Model file for the job. Use its own axes, mm. Give positions to 0.01 mm unless a question says otherwise; leave off trailing zeros. Loops run counter-clockwise (first coordinate to the right, second up) from the corner with the lowest first, then second, coordinate; pieces in that order, holes last. Notation, with made-up numbers: M 65.5,57.5 L 78.5,57.5 A31 cw 78.5,96.5 Z; hole C 46.5,30.5 d8. An arc over 180 degrees is marked long. Answer in a Markdown table with one row per item.
```python
from build123d import *

# Parameters (mm, degrees)
BOSS_EXTRUDE1_DEPTH = 9.3
SKETCH2_W           = 35
SKETCH2_H           = 6
BOSS_EXTRUDE2_DEPTH = 9.3


with BuildPart() as part:
    # Sketch1 → Boss-Extrude1 (new body)
    with BuildSketch(Plane.XY):
        Polygon((0, 0), (0, 42), (-10, 42), (-35, 2), (-35, 0), align=None)
    extrude(amount=-BOSS_EXTRUDE1_DEPTH)

    # Sketch2 → Boss-Extrude2 (add)
    with BuildSketch(Plane.XY):
        with Locations((-17.5, -3)):
            Rectangle(SKETCH2_W, SKETCH2_H)
    extrude(amount=-BOSS_EXTRUDE2_DEPTH)


solid = part.part
```
Q1. Saw through at A-A (z = -6.5). Give the cut face in (x, y).
Reported:
| item | result |
|---|---|
| outline | M -35,-6 L 0,-6 L 0,42 L -10,42 L -35,2 Z |
Q2. Drop flat-ended pins along their axis: pin 1 (4 mm diameter, centred on y = 31, z = -5.5, fed in from -X) (3 decimals); pin 2 (1.5 mm diameter, centred on x = -6, y = 16, fed in from +Z). Give the stop position or say it passes through.
Reported:
| item | result |
|---|---|
| pin 1 | x = -18.125 |
| pin 2 | z = 0 |
Q3. Probe probe 1 along X at (y, z) = (31, -4.75) (3 decimals); probe 2 along X at (y, z) = (37, -3.75) (3 decimals); probe 3 along Y at (x, z) = (-24.5, -4). List the from-to ranges inside material, lowest first.
Reported:
| item | result |
|---|---|
| probe 1 | -16.875 to 0 |
| probe 2 | -13.125 to 0 |
| probe 3 | -6 to 18.8 |
Q4. Saw through at C-C (y = 9). Give the cut face in (x, z) (3 decimals), and give its area (3 significant figures).
Reported:
| item | result |
|---|---|
| outline | M -30.625,-9.3 L 0,-9.3 L 0,0 L -30.625,0 Z |
| area | 285 mm² |
Q5. Saw through at B-B (x = -23). Give the cut face in (y, z).
Reported:
| item | result |
|---|---|
| outline | M -6,-9.3 L 21.2,-9.3 L 21.2,0 L -6,0 Z |
